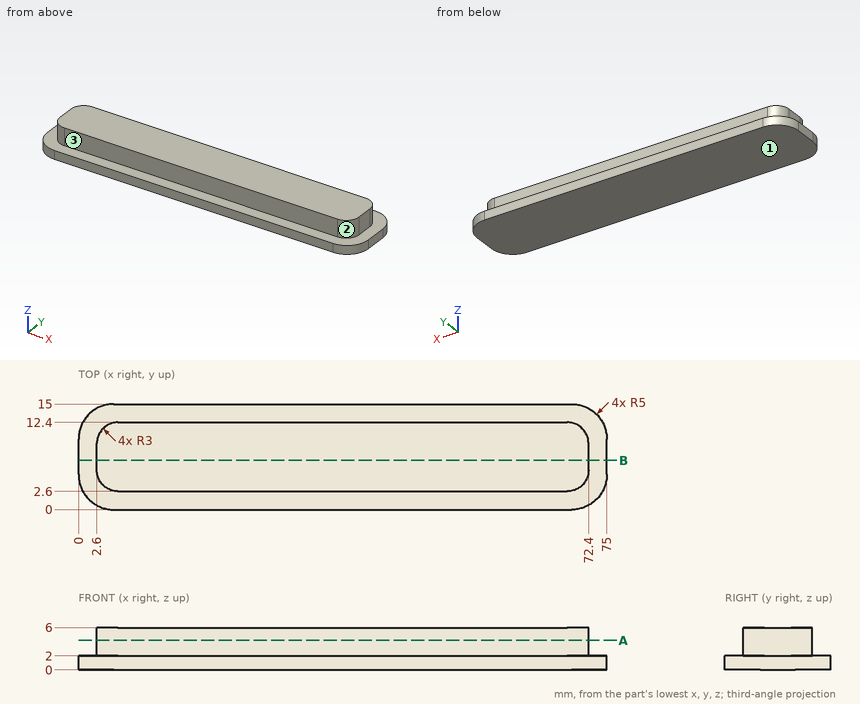
Verification items for this drawing (mm, ordinates from the low corner). A direction names the side the tool comes from. Round coordinates to 2 decimals unless told otherwise and drop trailing zeros. Order: outer loops, then holes, each group sorted by start corner. A loop starts at its lowest first (then second) coordinate and runs counter-clockwise, first axis right, second up. Notation, with made-up numbers: (89, 49) -> (147, 49) arc R24 ccw to (147, 62) -> close; hole circle Ø3 at (-5, -5.5). An arc over 180 degrees is marked (long way). Use one line per item in the form item = value.
1. Set-up check for the marked faces 1, 2 and 3: record each of +Z, -Z, +X, -X, +Y, -Y from which the full face is reachable in a straight line by a thin tool's end or side.
Working result:
face_1 = -Z, +X, -X, +Y, -Y
face_2 = +Z, +X, -Y
face_3 = +Z, +X, -X, -Y
2. Go/stop test with flat-tipped pins: pin 1 (3 mm diameter, centred on x = 31.5, z = 4.5, fed in from -Y); pin 2 (1 mm diameter, centred on y = 12.5, z = 1, fed in from -X); pin 3 (8 mm diameter, centred on x = 40.5, y = 2, fed in from +Z); pin 4 (1.1 mm diameter, centred on y = 6.5, z = 3, fed in from -X). Record where each tip stops, or that it passes through.
Working result:
pin_1 = 2.6
pin_2 = 0.42
pin_3 = 6
pin_4 = 2.6
3. Scan lines: line 1 along Y through (x, z) = (53.5, 2.55); line 2 along Z through (x, y) = (62, 1.5); line 3 along X through (y, z) = (8.5, 3.1). Record each from-to range of solid material in increasing order. Write a range as from..to.
Working result:
line_1 = 2.6..12.4
line_2 = 0..2
line_3 = 2.6..72.4
4. Cross-section at B-B, the plane y = 7. Enter the section's corners in (x, z), plus the area to 3 significant figures.
Working result:
outline = (0, 0) -> (75, 0) -> (75, 2) -> (72.4, 2) -> (72.4, 6) -> (2.6, 6) -> (2.6, 2) -> (0, 2) -> close
area = 429 mm^2
5. Cross-section at A-A, the plane z = 4.2. Enter the section's corners in (x, y), plus the area to 3 significant figures.
Working result:
outline = (2.6, 5.6) arc R3 ccw to (5.6, 2.6) -> (69.4, 2.6) arc R3 ccw to (72.4, 5.6) -> (72.4, 9.4) arc R3 ccw to (69.4, 12.4) -> (5.6, 12.4) arc R3 ccw to (2.6, 9.4) -> close
area = 676 mm^2
